Could you check a few things on this drawing? It's one solid part, dimensions in mm from its lowest x, y, z. A direction names the side the tool comes from. Give positions to 0.01 mm unless a question says otherwise; leave off trailing zeros. Order: outer loops, then holes, each group sorted by start corner. A loop starts at its lowest first (then second) coordinate and runs counter-clockwise, first axis right, second up.
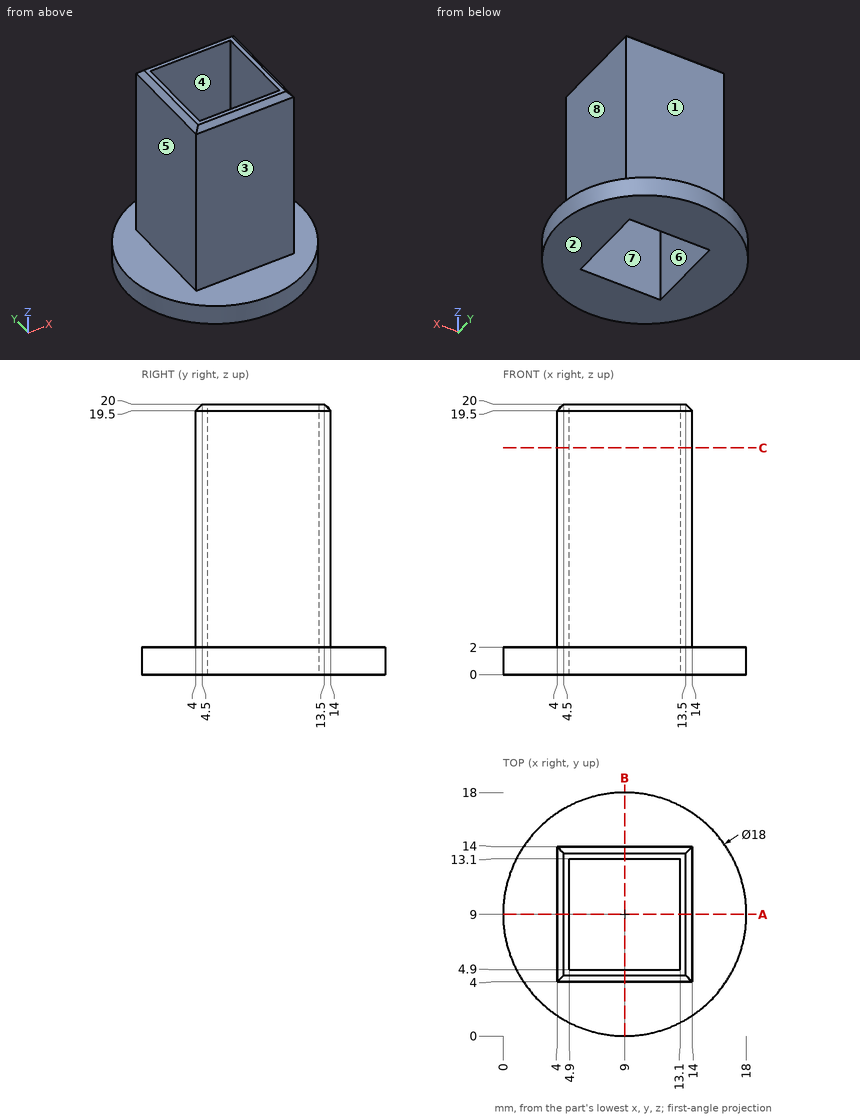
Item 1: Please list where these lines run through material, in increasing order: line 1 along X through (y, z) = (6.5, 16); line 2 along Z through (x, y) = (5.75, 16.75).
Findings:
line 1: x = 4 to 4.9, 13.1 to 14
line 2: z = 0 to 2
Item 2: We'd pull the mould along X, two halves only. Please class the marked faces 5, 6, 7 and 8: +X half, -X half, draft (parallel to the pull), parting line (faces both ways), or undercut.
Findings:
face 5: -X half
face 6: undercut
face 7: undercut
face 8: +X half
Item 3: For pin 1 (5 mm diameter, centred on x = 2.5, z = 14.5, fed in from +Y); pin 2 (6 mm diameter, centred on y = 9.5, z = 10.5, fed in from +X); pin 3 (9 mm diameter, centred on x = 7, z = 13, fed in from -Y), each with a flat end and sliding along its axis, tell me the tip position at first contact or that it passes through.
Findings:
pin 1: stops at y = 14
pin 2: stops at x = 14
pin 3: stops at y = 4
Item 4: For the marked faces 1, 2, 3 and 4, which set-ups out of +Z, -Z, +X, -X, +Y, -Y let a thin tool reach every point of the face, with its end or its side?
Findings:
face 1: +Z, +X, -X, +Y
face 2: -Z, +X, -X, +Y, -Y
face 3: +Z, +X, -X, -Y
face 4: +Z, -Z
Item 5: Imagine slicing it at C-C on z = 16.75. List the corners of the cut face in (x, y) for me, then the cut area to 3 significant figures.
Findings:
outline: (4, 4) - (14, 4) - (14, 14) - (4, 14) - close; hole (4.9, 4.9) - (13.1, 4.9) - (13.1, 13.1) - (4.9, 13.1) - close
area: 32.8 mm2
Item 6: Imagine slicing it at A-A on y = 9. List the corners of the cut face in (x, z) for me.
Findings:
outline: (0, 0) - (4.9, 0) - (4.9, 20) - (4.5, 20) - (4, 19.5) - (4, 2) - (0, 2) - close; (13.1, 0) - (18, 0) - (18, 2) - (14, 2) - (14, 19.5) - (13.5, 20) - (13.1, 20) - close
